Drawing for the job (mm, zero at the part's lowest x, y, z). Round coordinates to 2 decimals unless told otherwise and drop trailing zeros. Loops run counter-clockwise (first coordinate to the right, second up) from the corner with the lowest first, then second, coordinate; pieces in that order, holes last.
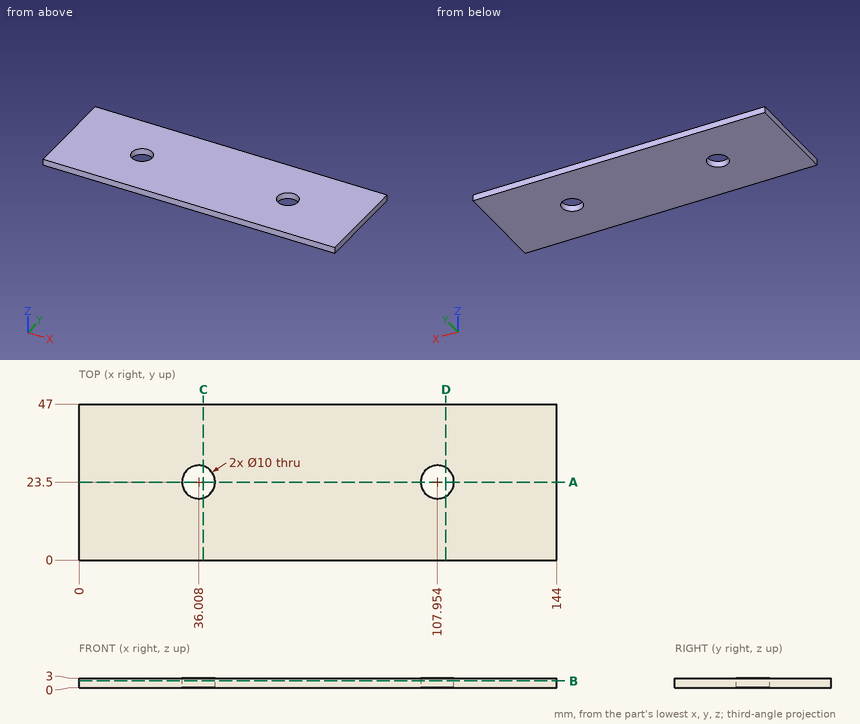
Q1. Probe line 1 (X direction, y = 23.5, z = 1.65); line 2 (X direction, y = 26.5, z = 2.7) (1 decimal); line 3 (Y direction, x = 37.5, z = 2.45). List the from-to ranges inside material, lowest first.
Q2. Slice it at C-C on x = 37.5. Give the cut face in (y, z).
Q3. Slice it at D-D on x = 110.5. Give the cut face in (y, z), plus the area to 3 significant figures.
Q4. Slice it at A-A on y = 23.5. Give the cut face in (x, z).
Q5. Flat gauge pin, fed straight in: P1, Ø3, axis at x = 123, y = 37.5, coming from the -Z side. Where does the tip first touch, or does it go through?
Q6. Slice it at B-B on z = 2.1. Give the cut face in (x, y).
Reply:
1. line 1: x = 0 to 31.01, 41.01 to 102.95, 112.95 to 144
1. line 2: x = 0 to 32, 40 to 104, 112 to 144
1. line 3: y = 0 to 18.73, 28.27 to 47
2. outline: (0, 0) - (18.73, 0) - (18.73, 3) - (0, 3) - close; (28.27, 0) - (47, 0) - (47, 3) - (28.27, 3) - close
3. outline: (0, 0) - (19.2, 0) - (19.2, 3) - (0, 3) - close; (27.8, 0) - (47, 0) - (47, 3) - (27.8, 3) - close
3. area: 115 mm2
4. outline: (0, 0) - (31.01, 0) - (31.01, 3) - (0, 3) - close; (41.01, 0) - (102.95, 0) - (102.95, 3) - (41.01, 3) - close; (112.95, 0) - (144, 0) - (144, 3) - (112.95, 3) - close
5. P1: stops at z = 0
6. outline: (0, 0) - (144, 0) - (144, 47) - (0, 47) - close; hole circle Ø10 at (36.01, 23.5); hole circle Ø10 at (107.95, 23.5)
